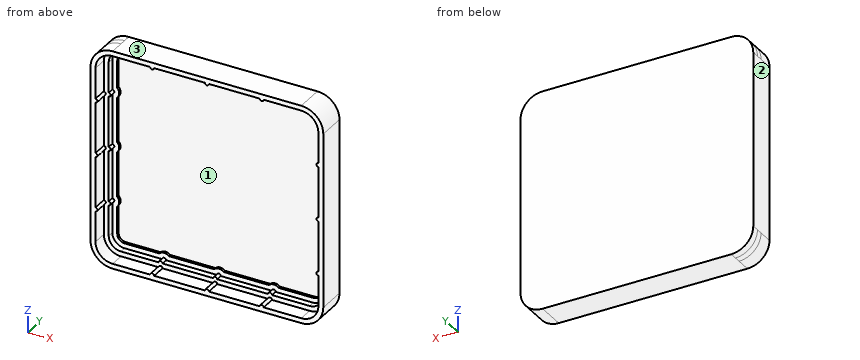
from build123d import *

# Parameters (mm, degrees)
BOSS_EXTRUDE1_DEPTH = 1.3
BOSS_EXTRUDE2_DEPTH = 1.5
SKETCH3_R           = 0.4
BOSS_EXTRUDE3_DEPTH = 1.3
BOSS_EXTRUDE4_DEPTH = 3
CUT_EXTRUDE1_DEPTH  = 0.5
SKETCH8_R           = 0.4
BOSS_EXTRUDE5_DEPTH = 3


with BuildPart() as part:
    # Sketch1 → Boss-Extrude1 (new body)
    with BuildSketch(Plane(origin=(0, 0, 0), x_dir=(1, 0, 0), z_dir=(0, 1, 0))):
        with BuildLine():
            Line((-19.250000047, -22.35), (19.25, -22.35))
            ThreePointArc((19.25, -22.35), (22.431980515, -21.031980515), (23.75, -17.85))
            Line((23.75, -17.85), (23.75, 17.85))
            ThreePointArc((23.75, 17.85), (22.431980515, 21.031980515), (19.25, 22.35))
            Line((19.25, 22.35), (-19.249999992, 22.35))
            ThreePointArc((-19.249999992, 22.35), (-22.431980512, 21.031980518), (-23.75, 17.85))
            Line((-23.75, 17.85), (-23.75, -17.85))
            ThreePointArc((-23.75, -17.85), (-22.431980532, -21.031980499), (-19.250000047, -22.35))
        make_face()
        with BuildLine():
            ThreePointArc((19.25, 20.35), (21.017766953, 19.617766953), (21.75, 17.85))
            Line((21.75, 17.85), (21.75, -17.85))
            ThreePointArc((21.75, -17.85), (21.017766953, -19.617766953), (19.25, -20.35))
            Line((19.25, -20.35), (-19.25, -20.35))
            ThreePointArc((-19.25, -20.35), (-21.017766953, -19.617766953), (-21.75, -17.85))
            Line((-21.75, -17.85), (-21.75, 17.85))
            ThreePointArc((-21.75, 17.85), (-21.017766953, 19.617766953), (-19.25, 20.35))
            Line((-19.25, 20.35), (19.25, 20.35))
        make_face(mode=Mode.SUBTRACT)
    extrude(amount=BOSS_EXTRUDE1_DEPTH)

    # Sketch2 → Boss-Extrude2 (add)
    with BuildSketch(Plane(origin=(0, 1.3, 0), x_dir=(1, 0, 0), z_dir=(0, 1, 0))):
        with BuildLine():
            Line((-19.25, -22.35), (19.25, -22.35))
            ThreePointArc((19.25, -22.35), (22.431980515, -21.031980515), (23.75, -17.85))
            Line((23.75, -17.85), (23.75, 17.85))
            ThreePointArc((23.75, 17.85), (22.431980515, 21.031980515), (19.25, 22.35))
            Line((19.25, 22.35), (-19.25, 22.35))
            ThreePointArc((-19.25, 22.35), (-22.431980515, 21.031980515), (-23.75, 17.85))
            Line((-23.75, 17.85), (-23.75, -17.85))
            ThreePointArc((-23.75, -17.85), (-22.431980515, -21.031980515), (-19.25, -22.35))
        make_face()
    extrude(amount=BOSS_EXTRUDE2_DEPTH)

    # Sketch3 → Boss-Extrude3 (add)
    with BuildSketch(Plane.XZ.offset(-1.3)):
        with Locations((-21.75, 11.175)):
            Circle(SKETCH3_R)
        with Locations((-21.75, 0)):
            Circle(SKETCH3_R)
        with Locations((-21.75, -11.175)):
            Circle(SKETCH3_R)
        with Locations((-11.175, -20.35)):
            Circle(SKETCH3_R)
        with Locations((11.175, -20.35)):
            Circle(SKETCH3_R)
        with Locations((21.75, -11.175)):
            Circle(SKETCH3_R)
        with Locations((21.75, 0)):
            Circle(SKETCH3_R)
        with Locations((21.75, 11.175)):
            Circle(SKETCH3_R)
        with Locations((11.175, 20.35)):
            Circle(SKETCH3_R)
        with Locations((0, 20.35)):
            Circle(SKETCH3_R)
        with Locations((-11.175, 20.35)):
            Circle(SKETCH3_R)
        with Locations((0, -20.35)):
            Circle(SKETCH3_R)
    extrude(amount=BOSS_EXTRUDE3_DEPTH)

    # Sketch4 → Boss-Extrude4 (add)
    with BuildSketch(Plane.XZ):
        with BuildLine():
            Line((19.25, 22.35), (-19.25, 22.35))
            ThreePointArc((-19.25, 22.35), (-22.431980515, 21.031980515), (-23.75, 17.85))
            Line((-23.75, 17.85), (-23.75, -17.85))
            ThreePointArc((-23.75, -17.85), (-22.431980515, -21.031980515), (-19.25, -22.35))
            Line((-19.25, -22.35), (19.25, -22.35))
            ThreePointArc((19.25, -22.35), (22.431980515, -21.031980515), (23.75, -17.85))
            Line((23.75, -17.85), (23.75, 17.85))
            ThreePointArc((23.75, 17.85), (22.431980515, 21.031980515), (19.25, 22.35))
        make_face()
        with BuildLine():
            Line((-22.75, 17.85), (-22.75, -17.85))
            ThreePointArc((-22.75, -17.85), (-21.724873734, -20.324873734), (-19.25, -21.35))
            Line((-19.25, -21.35), (19.25, -21.35))
            ThreePointArc((19.25, -21.35), (21.724873734, -20.324873734), (22.75, -17.85))
            Line((22.75, -17.85), (22.75, 17.85))
            ThreePointArc((22.75, 17.85), (21.724873734, 20.324873734), (19.25, 21.35))
            Line((19.25, 21.35), (-19.25, 21.35))
            ThreePointArc((-19.25, 21.35), (-21.724873734, 20.324873734), (-22.75, 17.85))
        make_face(mode=Mode.SUBTRACT)
    extrude(amount=BOSS_EXTRUDE4_DEPTH)

    # Sketch5 → Cut-Extrude1 (cut)
    with BuildSketch(Plane.XZ.offset(-1.3)):
        with BuildLine():
            Line((0.979795897, -19.35), (10.195204103, -19.35))
            ThreePointArc((10.195204103, -19.35), (11.175, -18.95), (12.154795897, -19.35))
            Line((12.154795897, -19.35), (19.25, -19.35))
            ThreePointArc((19.25, -19.35), (20.310660172, -18.910660172), (20.75, -17.85))
            Line((20.75, -17.85), (20.75, -12.154795897))
            ThreePointArc((20.75, -12.154795897), (20.35, -11.175), (20.75, -10.195204103))
            Line((20.75, -10.195204103), (20.75, -0.979795897))
            ThreePointArc((20.75, -0.979795897), (20.35, 0), (20.75, 0.979795897))
            Line((20.75, 0.979795897), (20.75, 10.195204103))
            ThreePointArc((20.75, 10.195204103), (20.35, 11.175), (20.75, 12.154795897))
            Line((20.75, 12.154795897), (20.75, 17.85))
            ThreePointArc((20.75, 17.85), (20.310660172, 18.910660172), (19.25, 19.35))
            Line((19.25, 19.35), (12.154795897, 19.35))
            ThreePointArc((12.154795897, 19.35), (11.175, 18.95), (10.195204103, 19.35))
            Line((10.195204103, 19.35), (0.979795897, 19.35))
            ThreePointArc((0.979795897, 19.35), (0, 18.95), (-0.979795897, 19.35))
            Line((-0.979795897, 19.35), (-10.195204103, 19.35))
            ThreePointArc((-10.195204103, 19.35), (-11.175, 18.95), (-12.154795897, 19.35))
            Line((-12.154795897, 19.35), (-19.25, 19.35))
            ThreePointArc((-19.25, 19.35), (-20.310660172, 18.910660172), (-20.75, 17.85))
            Line((-20.75, 17.85), (-20.75, 12.154795897))
            ThreePointArc((-20.75, 12.154795897), (-20.35, 11.175), (-20.75, 10.195204103))
            Line((-20.75, 10.195204103), (-20.75, 0.979795897))
            ThreePointArc((-20.75, 0.979795897), (-20.35, 0), (-20.75, -0.979795897))
            Line((-20.75, -0.979795897), (-20.75, -10.195204103))
            ThreePointArc((-20.75, -10.195204103), (-20.35, -11.175), (-20.75, -12.154795897))
            Line((-20.75, -12.154795897), (-20.75, -17.85))
            ThreePointArc((-20.75, -17.85), (-20.310660172, -18.910660172), (-19.25, -19.35))
            Line((-19.25, -19.35), (-12.154795897, -19.35))
            ThreePointArc((-12.154795897, -19.35), (-11.175, -18.95), (-10.195204103, -19.35))
            Line((-10.195204103, -19.35), (-0.979795897, -19.35))
            ThreePointArc((-0.979795897, -19.35), (0, -18.95), (0.979795897, -19.35))
        make_face()
    extrude(amount=-CUT_EXTRUDE1_DEPTH, mode=Mode.SUBTRACT)

    # Sketch8 → Boss-Extrude5 (add)
    with BuildSketch(Plane.XZ):
        with Locations((-11.175, 21.35)):
            Circle(SKETCH8_R)
        with Locations((0, 21.35)):
            Circle(SKETCH8_R)
        with Locations((11.175, 21.35)):
            Circle(SKETCH8_R)
        with Locations((22.75, 11.175)):
            Circle(SKETCH8_R)
        with Locations((-22.75, 11.175)):
            Circle(SKETCH8_R)
        with Locations((-22.75, 0)):
            Circle(SKETCH8_R)
        with Locations((22.75, 0)):
            Circle(SKETCH8_R)
        with Locations((22.75, -11.175)):
            Circle(SKETCH8_R)
        with Locations((11.175, -21.35)):
            Circle(SKETCH8_R)
        with Locations((0, -21.35)):
            Circle(SKETCH8_R)
        with Locations((-11.175, -21.35)):
            Circle(SKETCH8_R)
        with Locations((-22.75, -11.175)):
            Circle(SKETCH8_R)
    extrude(amount=BOSS_EXTRUDE5_DEPTH)


solid = part.part
Could you check a few things on this model? Use its own coordinates, in mm. Face numbers are marked on the shaded views. Round coordinates to 2 decimals unless told otherwise and drop trailing zeros. Write each loop counter-clockwise with the first axis right and the second up, starting at its lowest first coordinate (ties: lowest second). Pieces come first, ordered by that corner, then holes. Notation, with made-up numbers: (-4.5, 51) - (27.5, 51) arc R15 ccw to (27.5, 80) - close; hole circle Ø2 at (-0.75, -4.5). An arc over 180 degrees is marked (long way). Put each result on its own line as item: value. Start each with the question number.
(1) I want a section at A-A, the plane x = -8. Please give me the cut outline in (y, z), plus the area to 3 significant figures.
(2) Will this pin go through, and if not, where does the flat tip stop? pin 1 (1 mm diameter, centred on x = 0.5, z = -4, fed in from -Y).
(3) I want a section at B-B, the plane z = 16. Please give me the cut outline in (x, y).
(4) Thinking about a two-plate mould opening in Z: for the marked faces 1, 2 and 3, which applies, released by +Z, released by -Z, zero draft, split by the parting line, or undercut?
(5) I need wall thicknesses on probe 1 along X at (y, z) = (-2, -8.5); probe 2 along Z at (x, y) = (8, 1.1); probe 3 along Z at (x, y) = (-4, 1.5). Which ranges of each line are inside material? Lowest first, please.
Here are the results:
1. outline: (-3, -22.35) - (2.8, -22.35) - (2.8, 22.35) - (-3, 22.35) - (-3, 21.35) - (0, 21.35) - (0, 20.35) - (1.3, 20.35) - (1.3, 19.35) - (1.8, 19.35) - (1.8, -19.35) - (1.3, -19.35) - (1.3, -20.35) - (0, -20.35) - (0, -21.35) - (-3, -21.35) - close
1. area: 58.9 mm^2
2. pin 1: stops at y = 1.8
3. outline: (-23.75, -3) - (-22.75, -3) - (-22.75, 0) - (-21.75, 0) - (-21.75, 1.3) - (-20.75, 1.3) - (-20.75, 1.8) - (20.75, 1.8) - (20.75, 1.3) - (21.75, 1.3) - (21.75, 0) - (22.75, 0) - (22.75, -3) - (23.75, -3) - (23.75, 2.8) - (-23.75, 2.8) - close
4. face 1: undercut
4. face 2: zero draft
4. face 3: released by +Z
5. probe 1: x = -23.75 to -22.75, 22.75 to 23.75
5. probe 2: z = -22.35 to -20.35, 20.35 to 22.35
5. probe 3: z = -22.35 to -19.35, 19.35 to 22.35
